The figure shows three views and two pictorial views of one solid part (mm, origin at its lowest corner). Answer the questions. A direction names the side the tool comes from. Round coordinates to 2 decimals unless told otherwise and drop trailing zeros. Order: outer loops, then holes, each group sorted by start corner. A loop starts at its lowest first (then second) coordinate and runs counter-clockwise, first axis right, second up. Notation, with made-up numbers: (22, 85) - (54, 85) arc R32 cw to (54, 116) - close; hole circle Ø11 at (-40, 30.5). An arc over 180 degrees is marked (long way). Write item = value, one per line.
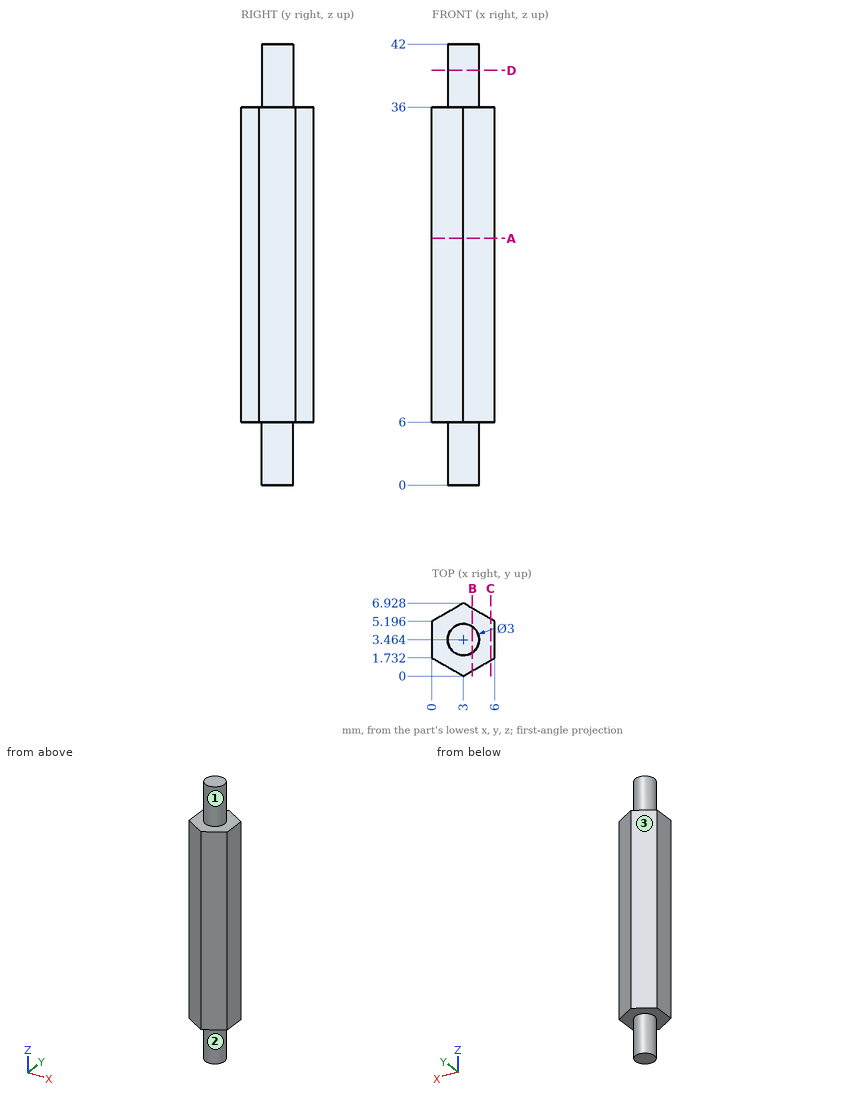
Q1. Section A-A on z = 23.5 is taken. Determine the outline of the cut face in (x, y).
Model answer:
outline = (0, 1.73) - (3, 0) - (6, 1.73) - (6, 5.2) - (3, 6.93) - (0, 5.2) - close
Q2. Section C-C on x = 5.6 is taken. Determine the outline of the cut face in (y, z), then the cut area to 3 significant figures.
Model answer:
outline = (1.5, 6) - (5.43, 6) - (5.43, 36) - (1.5, 36) - close
area = 118 mm^2
Q3. Section D-D on z = 39.5 is taken. Determine the outline of the cut face in (x, y).
Model answer:
outline = circle Ø3 at (3, 3.46)
Q4. For the marked faces 1, 2 and 3, determine the directions among +Z, -Z, +X, -X, +Y, -Y from which every point of the face is accessible in a straight line to the end or side of a thin tool.
Model answer:
face_1 = +Z
face_2 = -Z
face_3 = +Z, -Z, -X, +Y
Q5. Find the intervals of material crossed by line 1 (Z direction, x = 4.25, y = 4.5); line 2 (Y direction, x = 2.6, z = 10); line 3 (X direction, y = 1, z = 16.5), in increasing order. Write a range as from..to.
Model answer:
line_1 = 6..36
line_2 = 0.23..6.7
line_3 = 1.27..4.73
Q6. Section B-B on x = 3.85 is taken. Determine the outline of the cut face in (y, z).
Model answer:
outline = (0.49, 6) - (2.23, 6) - (2.23, 0) - (4.7, 0) - (4.7, 6) - (6.44, 6) - (6.44, 36) - (4.7, 36) - (4.7, 42) - (2.23, 42) - (2.23, 36) - (0.49, 36) - close
Q7. A flat-ended cylindrical pin translates along its axis: P1, Ø1, axis at x = 2, y = 5, coming from the +Z side. Find the tip coordinate at first contact, or state that the pin passes through.
Model answer:
P1 = 42
